Work out the finished part from the listing and answer in its coordinate system (mm). Face numbers are marked on the shaded views. A direction names the side the tool comes from. Round coordinates to 2 decimals unless told otherwise and drop trailing zeros. Order: outer loops, then holes, each group sorted by start corner. A loop starts at its lowest first (then second) coordinate and runs counter-clockwise, first axis right, second up. Notation, with made-up numbers: (-22.5, 41) - (4.5, 41) arc R5 ccw to (4.5, 47) - close; hole circle Ø8 at (16, 13). An arc over 180 degrees is marked (long way). Answer in a Markdown table with one row per item.
from build123d import *

# Parameters (mm, degrees)
SKETCH1_W           = 13
SKETCH1_H           = 20
BOSS_EXTRUDE1_DEPTH = 3
SKETCH2_W           = 3
SKETCH2_H           = 1.5
CUT_EXTRUDE1_DEPTH  = 3
SKETCH3_W           = 3
SKETCH3_H           = 1.5
CUT_EXTRUDE2_DEPTH  = 3
SKETCH5_W           = 5
SKETCH5_H           = 3
CUT_EXTRUDE6_DEPTH  = 3
SKETCH6_W           = 3
SKETCH6_H           = 1.5
CUT_EXTRUDE7_DEPTH  = 10


with BuildPart() as part:
    # Sketch1 → Boss-Extrude1 (new body)
    with BuildSketch(Plane.XY):
        with Locations((0, 4.633458647)):
            Rectangle(SKETCH1_W, SKETCH1_H)
    extrude(amount=BOSS_EXTRUDE1_DEPTH)

    # Sketch2 → Cut-Extrude1 (cut)
    with BuildSketch(Plane.XY.offset(3)):
        with Locations((-5, 11.883458647)):
            Rectangle(SKETCH2_W, SKETCH2_H)
        with Locations((-5, 7.383458647)):
            Rectangle(SKETCH2_W, SKETCH2_H)
    extrude(amount=-CUT_EXTRUDE1_DEPTH, mode=Mode.SUBTRACT)

    # Sketch3 → Cut-Extrude2 (cut)
    with BuildSketch(Plane.XY.offset(3)):
        with Locations((5, 11.883458647)):
            Rectangle(SKETCH3_W, SKETCH3_H)
        with Locations((5, 7.383458647)):
            Rectangle(SKETCH3_W, SKETCH3_H)
    extrude(amount=-CUT_EXTRUDE2_DEPTH, mode=Mode.SUBTRACT)

    # Sketch5 → Cut-Extrude6 (cut)
    with BuildSketch(Plane.XY.offset(3)):
        with Locations((0, 13.133458647)):
            Rectangle(SKETCH5_W, SKETCH5_H)
    extrude(amount=-CUT_EXTRUDE6_DEPTH, mode=Mode.SUBTRACT)

    # Sketch6 → Cut-Extrude7 (cut)
    with BuildSketch(Plane.XY.offset(3)):
        with Locations((-5, 2.883458647)):
            Rectangle(SKETCH6_W, SKETCH6_H)
        with Locations((-5, -1.616541353)):
            Rectangle(SKETCH6_W, SKETCH6_H)
        with Locations((5, 2.883458647)):
            Rectangle(SKETCH6_W, SKETCH6_H)
        with Locations((5, -1.616541353)):
            Rectangle(SKETCH6_W, SKETCH6_H)
    extrude(amount=-CUT_EXTRUDE7_DEPTH, mode=Mode.SUBTRACT)


solid = part.part
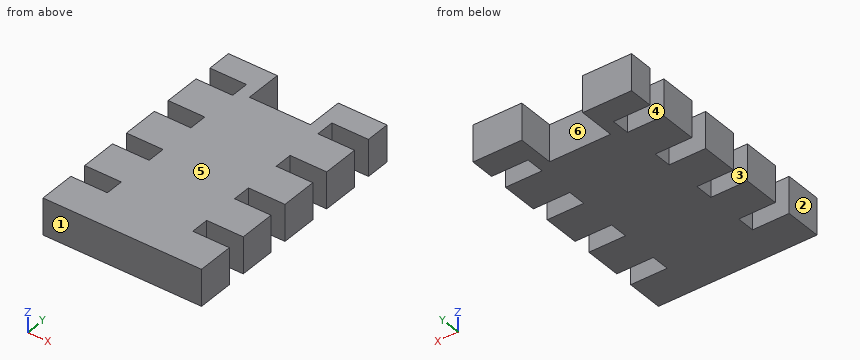
1) Which of the six approach directions +Z, -Z, +X, -X, +Y, -Y give full straight-line access (tool end or side, diameter ignored) to the marked faces 5 and 6?
Filled in:
| item | result |
|---|---|
| face 5 | +Z, +X, -X, +Y, -Y |
| face 6 | +Z, -Z, +Y |
2) The mould has two halves that part along Y. Classify the marked faces 1, 2, 3 and 4: released by +Y, released by -Y, zero draft, split by the parting line, or undercut.
Filled in:
| item | result |
|---|---|
| face 1 | released by -Y |
| face 2 | zero draft |
| face 3 | undercut |
| face 4 | undercut |
3) Find the intervals of material crossed by probe 1 along Y at (x, z) = (4, 1.7); probe 2 along X at (y, z) = (12.5, 0.35); probe 3 along Y at (x, z) = (-2, 2.6), in increasing order. Write a range as from..to.
Filled in:
| item | result |
|---|---|
| probe 1 | y = -5.37..-2.37, -0.87..2.13, 3.63..6.63, 8.13..11.13, 12.63..14.63 |
| probe 2 | x = -3.5..-2.5, 2.5..3.5 |
| probe 3 | y = -5.37..11.63 |
4) Find section C-C, the plane x = -0.25. Give the vertices of the cut face in (y, z).
Filled in:
| item | result |
|---|---|
| outline | (-5.37, 0) - (11.63, 0) - (11.63, 3) - (-5.37, 3) - close |
5) Find section A-A, the plane x = -5. Give the vertices of the cut face in (y, z).
Filled in:
| item | result |
|---|---|
| outline | (-5.37, 0) - (-2.37, 0) - (-2.37, 3) - (-5.37, 3) - close; (-0.87, 0) - (2.13, 0) - (2.13, 3) - (-0.87, 3) - close; (3.63, 0) - (6.63, 0) - (6.63, 3) - (3.63, 3) - close; (8.13, 0) - (11.13, 0) - (11.13, 3) - (8.13, 3) - close; (12.63, 0) - (14.63, 0) - (14.63, 3) - (12.63, 3) - close |
6) Find section B-B, the plane y = -2. Give the vertices of the cut face in (x, z), then the cut area to 3 significant figures.
Filled in:
| item | result |
|---|---|
| outline | (-3.5, 0) - (3.5, 0) - (3.5, 3) - (-3.5, 3) - close |
| area | 21.0 mm^2 |
7) Each of these flat-tipped pins is pushed along its axis until it touches: pin 1 (0.8 mm diameter, centred on y = 7.5, z = 2, fed in from -X); pin 2 (1.2 mm diameter, centred on y = 12, z = 1, fed in from +X). Where does it stop, or does it pass through?
Filled in:
| item | result |
|---|---|
| pin 1 | stops at x = -3.5 |
| pin 2 | stops at x = 3.5 |
